CAD build for the part. Positions are in the model's coordinates, mm. Face numbers are marked on the shaded views. A direction names the side the tool comes from. Round coordinates to 2 decimals unless told otherwise and drop trailing zeros. Loops run counter-clockwise (first coordinate to the right, second up) from the corner with the lowest first, then second, coordinate; pieces in that order, holes last. Notation, with made-up numbers: M 9,50 L 57,50 A31 ccw 57,87 Z; hole C -10,-5.75 d4. An arc over 180 degrees is marked long. Use one line per item in the form item = value.
from build123d import *

# Parameters (mm, degrees)
F0_R        = 40
F0_R_2      = 5
F1_DEPTH    = 15
F4_R        = 12.5
F5_DEPTH    = 12
F6_T6_ANGLE = 90
F6_T8_ANGLE = 270


# Not quite as in the source:
# - a fillet or chamfer that OpenCascade refuses, or shapes differently, is made with other operations: its cross-section is extruded or revolved along the edge and cut away or added


with BuildPart() as f1:
    # F0 (on Top) → F1 (new body)
    with BuildSketch(Plane.XY):
        Circle(F0_R)
        Circle(F0_R_2, mode=Mode.SUBTRACT)
    extrude(amount=F1_DEPTH)

    # F2 (on Right) → F3 (revolve, cut)
    with BuildSketch(Plane.YZ):
        Polygon((-30, 0), (0, 0), (0, 5), align=None)
    revolve(axis=Axis((0, 0, -3.8595963269), (0, 0, -1)), mode=Mode.SUBTRACT)

    # F4 (on Top) → F5 (cut)
    with BuildSketch(Plane.XY):
        Circle(F4_R)
    extrude(amount=F5_DEPTH, mode=Mode.SUBTRACT)

    # F6: chamfer of 0.5 on 6 edges, made by hand

    # F6_s1 → F6_t2 (revolve, cut)
    with BuildSketch(Plane.XZ):
        Polygon((40, 14.5), (39.5, 15), (40, 15), align=None)
    revolve(axis=Axis((0, 0, 15), (0, 0, 1)), mode=Mode.SUBTRACT)

    # F6_s3 → F6_t4 (revolve, cut)
    with BuildSketch(Plane.XZ):
        Polygon((40, 0.5), (39.5, 0), (40, 0), align=None)
    revolve(axis=Axis((0, 0, 0), (0, 0, 1)), mode=Mode.SUBTRACT)

    # F6_s5 → F6_t6 (revolve, cut)
    with BuildSketch(Plane.XZ):
        Polygon((12.9178005063, 2.8470332489), (12.5, 3.3402302109), (12.5, 2.9166666667), align=None)
    revolve(axis=Axis((0, 0, 2.9166666667), (0, 0, -1)), revolution_arc=F6_T6_ANGLE, mode=Mode.SUBTRACT)

    # F6_s7 → F6_t8 (revolve, cut)
    with BuildSketch(Plane.YZ):
        Polygon((-12.9178005063, 2.8470332489), (-12.5, 3.3402302109), (-12.5, 2.9166666667), align=None)
    revolve(axis=Axis((0, 0, 2.9166666667), (0, 0, -1)), revolution_arc=F6_T8_ANGLE, mode=Mode.SUBTRACT)

    # F6_s9 → F6_t10 (revolve, cut)
    with BuildSketch(Plane.XZ):
        Polygon((5, 12.5), (5.5, 12), (5, 12), align=None)
    revolve(axis=Axis((0, 0, 12), (0, 0, -1)), mode=Mode.SUBTRACT)

    # F6_s11 → F6_t12 (revolve, cut)
    with BuildSketch(Plane.XZ):
        Polygon((5.5, 15), (5, 14.5), (5, 15), align=None)
    revolve(axis=Axis((0, 0, 15), (0, 0, 1)), mode=Mode.SUBTRACT)


solid = f1.part
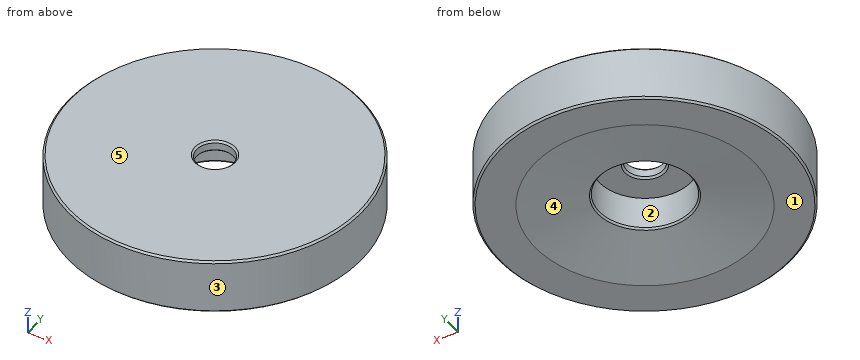
1. Probe line 1 along Y through (x, z) = (0, 13.65); line 2 along Y through (x, z) = (0, 8.75); line 3 along Z through (x, y) = (6, -23). List the from-to ranges inside material, lowest first. Write a range as from..to.
Completed:
line_1 = -40..-5, 5..40
line_2 = -40..-12.5, 12.5..40
line_3 = 1.04..15
2. Tool access for the marked faces 1 and 2: list every direction of +Z, -Z, +X, -X, +Y, -Y with a clear straight run to the whole face (end or side of a thin tool).
Completed:
face_1 = -Z, +X, -X, +Y, -Y
face_2 = -Z
3. Drop flat-ended pins along their axis: P1, Ø8, axis at x = 16.5, z = 1.5, coming from the +Y side; P2, Ø1.5, axis at x = 31.5, z = 10, coming from the +Y side; P3, Ø2, axis at x = -20.5, z = 4.5, coming from the -Y side. Give the stop position or say it passes through.
Completed:
P1 = 38
P2 = 25.58
P3 = -34.92
4. Cut at C-C on z = 8.75. Write the cut outline in (x, y), and give its area (3 significant figures).
Completed:
outline = C 0,0 d80; hole C 0,0 d25
area = 4,540 mm2
5. Cut at A-A on x = 0. Write the cut outline in (y, z), and give its area (3 significant figures).
Completed:
outline = M -40,0.5 L -39.5,0 L -30,0 L -12.92,2.85 L -12.5,3.34 L -12.5,12 L -5.5,12 L -5,12.5 L -5,14.5 L -5.5,15 L -39.5,15 L -40,14.5 Z; M 5,12.5 L 5.5,12 L 12.5,12 L 12.5,3.34 L 12.92,2.85 L 30,0 L 39.5,0 L 40,0.5 L 40,14.5 L 39.5,15 L 5.5,15 L 5,14.5 Z
area = 818 mm2
6. Pull direction Y, two halves, no side cores. Call the marked faces 3, 4 and 5: +Y half, -Y half, draft (parallel to the pull), parting line (faces both ways), or undercut.
Completed:
face_3 = parting line
face_4 = undercut
face_5 = draft
